```python
from build123d import *

# Parameters (mm, degrees)
SKETCH_R        = 25
PAD_DEPTH       = 15
PAD001_DEPTH    = 10
PAD001_FACE2_R  = 25
POCKET_DEPTH    = 13
POCKET001_DEPTH = 5
FILLET_R        = 1


with BuildPart() as part:
    # Sketch → Pad (new body)
    with BuildSketch(Plane.XY):
        Circle(SKETCH_R)
    extrude(amount=PAD_DEPTH)

    # Sketch001 (on Face3 of Pad) → Pad001 (join)
    with BuildSketch(Plane.XY.offset(15)):
        with BuildLine():
            ThreePointArc((2.575, 1.857418), (-3.175, 0), (2.575, -1.857418))
            Line((2.575, 1.857418), (2.575, -1.857418))
        make_face()
    extrude(amount=PAD001_DEPTH)

    # Pad001 Face2 → Pocket (cut)
    with BuildSketch(Plane(origin=(0, 0, 0), x_dir=(0, -1, 0), z_dir=(0, 0, -1))):
        Circle(PAD001_FACE2_R)
    extrude(amount=-POCKET_DEPTH, mode=Mode.SUBTRACT)

    # Pocket Face6 → Pocket001 (cut)
    with BuildSketch(Plane(origin=(-0.141681, 0, 25), x_dir=(0, 1, 0), z_dir=(0, 0, 1))):
        with BuildLine():
            ThreePointArc((1.857418, -2.716681), (0, 3.033319), (-1.857418, -2.716681))
            Line((-1.857418, -2.716681), (1.857418, -2.716681))
        make_face()
    extrude(amount=-POCKET001_DEPTH, mode=Mode.SUBTRACT)

    # Fillet
    fillet_edges = [part.edges().sort_by_distance(p)[0] for p in [
        (-25, 0, 13),
    ]]
    fillet(fillet_edges, radius=FILLET_R)


solid = part.part
```
Build history of the part. All positions in model axes, mm. A direction names the side the tool comes from. Give positions to 0.01 mm unless a question says otherwise; leave off trailing zeros. Loops run counter-clockwise (first coordinate to the right, second up) from the corner with the lowest first, then second, coordinate; pieces in that order, holes last.
Item 1: Drill centre lines: line 1 (Z direction, x = 15.5, y = -10); line 2 (Y direction, x = -20.5, z = 13.5); line 3 (Y direction, x = 4, z = 13.5). Where is each one in solid material? Low to high.
Answers follow:
line 1: z = 13 to 15
line 2: y = -14.07 to 14.07
line 3: y = -24.54 to 24.54
Item 2: Slice it at C-C, the plane z = 16.5. List the corners of the cut face in (x, y) (3 decimals).
Answers follow:
outline: (2.575, -1.857) - (2.575, 1.857) arc R3.175 ccw (long way) to start
Item 3: Which spindle directions (+Z, -Z, +X, -X, +Y, -Y) get a long thin tool onto all of the face, cutting with end or side? Do faces 1 (the face through (2.575, 0, 17)), 2 (the face through (-3.173, 0.112, 17.465)), 3 (the face through (0, 0, 20)). Say none if no direction does.
Answers follow:
face 1: +Z, +X, +Y, -Y
face 2: +Z
face 3: +Z, +X, -X, +Y, -Y
Item 4: Slice it at A-A, the plane y = 0. List the corners of the cut face in (x, z) (3 decimals), and give its area (3 significant figures).
Answers follow:
outline: (-25, 14) arc R1 ccw to (-24, 13) - (24, 13) arc R1 ccw to (25, 14) - (25, 15) - (2.575, 15) - (2.575, 20) - (-3.175, 20) - (-3.175, 15) - (-25, 15) - close
area: 128 mm2
Item 5: Flat gauge pins, fed straight in: pin 1 (1.1 mm diameter, centred on y = 0, z = 18.5, fed in from +X) (3 decimals); pin 2 (15 mm diameter, centred on x = -8, y = 12, fed in from +Z). Where does each tip first touch, or does it go through?
Answers follow:
pin 1: stops at x = 2.575
pin 2: stops at z = 15
Item 6: Slice it at B-B, the plane x = 0. List the corners of the cut face in (y, z) (3 decimals).
Answers follow:
outline: (-25, 14) arc R1 ccw to (-24, 13) - (24, 13) arc R1 ccw to (25, 14) - (25, 15) - (3.175, 15) - (3.175, 20) - (-3.175, 20) - (-3.175, 15) - (-25, 15) - close
